The model under review builds one solid part; all positions refer to its coordinate system, in mm. A direction names the side the tool comes from. Give positions to 0.01 mm unless a question says otherwise; leave off trailing zeros. Loops run counter-clockwise (first coordinate to the right, second up) from the corner with the lowest first, then second, coordinate; pieces in that order, holes last. Notation, with made-up numbers: M 44,28.25 L 66,28.25 A21 cw 66,47.25 Z; hole C 86.25,49.5 d1. An arc over 180 degrees is marked long. Write item = value, one per line. Start each with the question number.
1. We need section A-A on y = 85.25. Give the boundary of the cut face in (x, z), then the cut area to 3 significant figures.
2. We need section C-C on y = 77.5. Give the boundary of the cut face in (x, z).
3. We need section B-B on z = 12.25. Give the boundary of the cut face in (x, y), then the cut area to 3 significant figures.
4. We need section D-D on x = 6.5. Give the boundary of the cut face in (y, z).
5. Draft analysis for pull direction Y (two halves, no side actions). For faces 1 (the face through (-6.16, 59.66, 15.14)), 2 (the face through (-15.358, 47.727, 1.479)), 3 (the face through (6, 75, 16)), state which applies: pulls with the +Y half, pulls with the -Y half, needs draft (parallel to the pull), parting line crosses it, or undercut.
6. For faces 4 (the face through (6.16, 83.54, 12.63)), 5 (the face through (0, 60, 1)), 6 (the face through (-6, 58.761, 8)), list the 3-axis set-ups (+Z, -Z, +X, -X, +Y, -Y) from which the entire face can be reached by the end or side of a thin tool; tool diameter is ignored.
7. Wall thickness on line 1 along Z through (x, y) = (6.5, 85.25); line 2 along X through (y, z) = (71, 5); line 3 along Y through (x, z) = (5.8, 12.25): over which ranges is each line inside the solid? List them lowest first. Write a range as from..to.
8. For pin 1 (5 mm diameter, centred on y = 66, z = 13, fed in from +X); pin 2 (10 mm diameter, centred on x = 8.5, z = 13, fed in from -Y); pin 3 (1.5 mm diameter, centred on y = 76.5, z = 14, fed in from -X), all flat-tipped, find the tip position at first contact; note any pin that passes through.
from build123d import *

# Parameters (mm, degrees)
SKETCH2_R           = 5
SKETCH2_R_2         = 2.75
SKETCH2_W           = 2
SKETCH2_H           = 30
BOSS_EXTRUDE1_DEPTH = 3
SKETCH3_W           = 2
SKETCH3_H           = 31.239003023
BOSS_EXTRUDE2_DEPTH = 13
SKETCH4_W           = 2
SKETCH4_H           = 29.7
BOSS_EXTRUDE3_DEPTH = 2
SKETCH5_R           = 1.75
CUT_EXTRUDE1_DEPTH  = 96.357865433
FILLET1_R           = 3


with BuildPart() as part:
    # Sketch2 → Boss-Extrude1 (new body)
    # profile 1 of 13: a face of its own
    with BuildSketch(Plane.XY):
        with BuildLine():
            Line((0, 55), (-5.15, 55))
            Line((-5.15, 55), (-7.15, 55))
            Line((-7.15, 55), (-7.15, 58.760996977))
            ThreePointArc((-7.15, 58.760996977), (-14.633199965, 54.158827301), (-19.615384615, 46.923076923))
            ThreePointArc((-19.615384615, 46.923076923), (-14.019419324, 49.902903378), (-10, 45))
            ThreePointArc((-10, 45), (-7.071067812, 52.071067812), (0, 55))
        make_face()
    # profile 2 of 13: a face of its own
    with BuildSketch(Plane.XY):
        with Locations((-15, 45)):
            Circle(SKETCH2_R)
        with Locations((-15, 45)):
            Circle(SKETCH2_R_2, mode=Mode.SUBTRACT)
    # profile 3 of 13: a face of its own
    with BuildSketch(Plane.XY):
        with BuildLine():
            Line((7.15, 55), (5.15, 55))
            Line((5.15, 55), (0, 55))
            ThreePointArc((0, 55), (7.071067812, 52.071067812), (10, 45))
            ThreePointArc((10, 45), (14.019419324, 49.902903378), (19.615384615, 46.923076923))
            ThreePointArc((19.615384615, 46.923076923), (14.633199965, 54.158827301), (7.15, 58.760996977))
            Line((7.15, 58.760996977), (7.15, 55))
        make_face()
    # profile 4 of 13: a face of its own
    with BuildSketch(Plane.XY):
        with Locations((15, 45)):
            Circle(SKETCH2_R)
        with Locations((15, 45)):
            Circle(SKETCH2_R_2, mode=Mode.SUBTRACT)
    # profile 5 of 13: a face of its own
    with BuildSketch(Plane.XY):
        with BuildLine():
            ThreePointArc((5.15, 59.366498248), (2.594408626, 59.841029939), (0, 60))
            ThreePointArc((0, 60), (-2.594408626, 59.841029939), (-5.15, 59.366498248))
            Line((-5.15, 59.366498248), (-5.15, 55))
            Line((-5.15, 55), (0, 55))
            Line((0, 55), (5.15, 55))
            Line((5.15, 55), (5.15, 59.366498248))
        make_face()
    # profile 6 of 13: a face of its own
    with BuildSketch(Plane.XY):
        with BuildLine():
            ThreePointArc((7.15, 58.760996977), (6.157447356, 59.088346591), (5.15, 59.366498248))
            Line((5.15, 59.366498248), (5.15, 55))
            Line((5.15, 55), (7.15, 55))
            Line((7.15, 55), (7.15, 58.760996977))
        make_face()
    # profile 7 of 13: a face of its own
    with BuildSketch(Plane.XY):
        with BuildLine():
            Line((-5.15, 55), (-5.15, 59.366498248))
            ThreePointArc((-5.15, 59.366498248), (-6.157447356, 59.088346591), (-7.15, 58.760996977))
            Line((-7.15, 58.760996977), (-7.15, 55))
            Line((-7.15, 55), (-5.15, 55))
        make_face()
    # profile 8 of 13: a face of its own
    with BuildSketch(Plane.XY):
        with Locations((-6.15, 75)):
            Rectangle(SKETCH2_W, SKETCH2_H)
    # profile 9 of 13: a face of its own
    with BuildSketch(Plane.XY):
        with BuildLine():
            Line((-5.15, 59.366498248), (-5.15, 60))
            Line((-5.15, 60), (-7.15, 60))
            Line((-7.15, 60), (-7.15, 58.760996977))
            ThreePointArc((-7.15, 58.760996977), (-6.157447356, 59.088346591), (-5.15, 59.366498248))
        make_face()
    # profile 10 of 13: a face of its own
    with BuildSketch(Plane.XY):
        with BuildLine():
            ThreePointArc((-5.15, 59.366498248), (-2.594408626, 59.841029939), (0, 60))
            Line((0, 60), (-5.15, 60))
            Line((-5.15, 60), (-5.15, 59.366498248))
        make_face()
    # profile 11 of 13: a face of its own
    with BuildSketch(Plane.XY):
        with BuildLine():
            Line((5.15, 60), (0, 60))
            ThreePointArc((0, 60), (2.594408626, 59.841029939), (5.15, 59.366498248))
            Line((5.15, 59.366498248), (5.15, 60))
        make_face()
    # profile 12 of 13: a face of its own
    with BuildSketch(Plane.XY):
        with BuildLine():
            Line((7.15, 60), (5.15, 60))
            Line((5.15, 60), (5.15, 59.366498248))
            ThreePointArc((5.15, 59.366498248), (6.157447356, 59.088346591), (7.15, 58.760996977))
            Line((7.15, 58.760996977), (7.15, 60))
        make_face()
    # profile 13 of 13: a face of its own
    with BuildSketch(Plane.XY):
        with Locations((6.15, 75)):
            Rectangle(SKETCH2_W, SKETCH2_H)
    extrude(amount=BOSS_EXTRUDE1_DEPTH)

    # Sketch3 → Boss-Extrude2 (add)
    with BuildSketch(Plane.XY.offset(3)):
        with Locations((-6.15, 74.380498488)):
            Rectangle(SKETCH3_W, SKETCH3_H)
        with Locations((6.15, 74.380498488)):
            Rectangle(SKETCH3_W, SKETCH3_H)
    extrude(amount=BOSS_EXTRUDE2_DEPTH)

    # Sketch4 → Boss-Extrude3 (add)
    with BuildSketch(Plane(origin=(0, 0, 0), x_dir=(-1, 0, 0), z_dir=(0, 0, -1))):
        with Locations((-6.15, 75.15)):
            Rectangle(SKETCH4_W, SKETCH4_H)
        with Locations((6.15, 75.15)):
            Rectangle(SKETCH4_W, SKETCH4_H)
    extrude(amount=BOSS_EXTRUDE3_DEPTH)

    # Sketch5 → Cut-Extrude1 (cut, through all)
    with BuildSketch(Plane(origin=(7.15, 0, 0), x_dir=(0, 0, -1), z_dir=(1, 0, 0))):
        with Locations((-1.75, 62.75)):
            Circle(SKETCH5_R)
        with Locations((-12.25, 85.25)):
            Circle(SKETCH5_R)
    extrude(amount=-CUT_EXTRUDE1_DEPTH, mode=Mode.SUBTRACT)

    # Fillet1
    # the kernel refuses this fillet: 3 mm, written as the material it takes off along each edge
    with BuildSketch(Plane(origin=(1.921067812, 60.3, -2), x_dir=(0, 0, 1), z_dir=(-1, 0, 0))) as fillet1_piece_1:
        with BuildLine():
            CenterArc((3, 2.828427125), FILLET1_R, 180, 70.528779366)
            Line((0, 2.828427125), (-0.06, 2.828427125))
            Line((-0.06, 2.828427125), (-0.06, 0))
            Line((-0.06, 0), (0, -0.06))
            ThreePointArc((0, -0.06), (1, -0.06), (1.98, -0.056568542))
            Line((1.98, -0.056568542), (2, 0))
        make_face()
    extrude(amount=16.142135624, mode=Mode.SUBTRACT)
    with BuildSketch(Plane(origin=(-1.921067812, 60.3, -2), x_dir=(0, 0, 1), z_dir=(1, 0, 0))) as fillet1_piece_2:
        with BuildLine():
            CenterArc((3, -2.828427125), FILLET1_R, 109.471220634, 70.528779366)
            Line((0, -2.828427125), (-0.06, -2.828427125))
            Line((-0.06, -2.828427125), (-0.06, 0))
            Line((-0.06, 0), (0, 0.06))
            ThreePointArc((0, 0.06), (1, 0.06), (1.98, 0.056568542))
            Line((1.98, 0.056568542), (2, 0))
        make_face()
    extrude(amount=16.142135624, mode=Mode.SUBTRACT)
    with BuildSketch(Plane(origin=(14.65, 58.760996977, 16), x_dir=(0, 0, -1), z_dir=(-1, 0, 0)), Plane(origin=(14.65, 90, -2), x_dir=(0, 0, 1), z_dir=(-1, 0, 0)), Plane(origin=(-14.65, 90, -2), x_dir=(0, -1, 0), z_dir=(1, 0, 0)), Plane(origin=(-2.35, 90, 16), x_dir=(0, 0, -1), z_dir=(1, 0, 0)), Plane(origin=(2.35, 90, 16), x_dir=(0, -1, 0), z_dir=(-1, 0, 0))) as fillet1_piece_3:
        with BuildLine():
            CenterArc((FILLET1_R, -FILLET1_R), FILLET1_R, 90, 90)
            Line((0, -FILLET1_R), (-FILLET1_R * 0.02, -FILLET1_R))
            Line((-FILLET1_R * 0.02, -FILLET1_R), (-FILLET1_R * 0.02, FILLET1_R * 0.02))
            Line((-FILLET1_R * 0.02, FILLET1_R * 0.02), (FILLET1_R, FILLET1_R * 0.02))
            Line((FILLET1_R, FILLET1_R * 0.02), (FILLET1_R, 0))
        make_face()
    extrude(amount=17, mode=Mode.SUBTRACT)
    with BuildSketch(Plane(origin=(-14.65, 58.760996977, 16), x_dir=(0, 0, -1), z_dir=(1, 0, 0))) as fillet1_piece_4:
        with BuildLine():
            CenterArc((FILLET1_R, FILLET1_R), FILLET1_R, 180, 90)
            Line((0, FILLET1_R), (-FILLET1_R * 0.02, FILLET1_R))
            Line((-FILLET1_R * 0.02, FILLET1_R), (-FILLET1_R * 0.02, -FILLET1_R * 0.02))
            Line((-FILLET1_R * 0.02, -FILLET1_R * 0.02), (FILLET1_R, -FILLET1_R * 0.02))
            Line((FILLET1_R, -FILLET1_R * 0.02), (FILLET1_R, 0))
        make_face()
    extrude(amount=17, mode=Mode.SUBTRACT)


solid = part.part
Final values:
q1.outline = M -7.15,-2 L -5.15,-2 L -5.15,10.5 L -7.15,10.5 Z; M -7.15,14 L -5.15,14 L -5.15,16 L -7.15,16 Z; M 5.15,-2 L 7.15,-2 L 7.15,10.5 L 5.15,10.5 Z; M 5.15,14 L 7.15,14 L 7.15,16 L 5.15,16 Z
q1.area = 58.0 mm²
q2.outline = M -7.15,-2 L -5.15,-2 L -5.15,16 L -7.15,16 Z; M 5.15,-2 L 7.15,-2 L 7.15,16 L 5.15,16 Z
q3.outline = M -7.15,58.76 L -5.15,58.76 L -5.15,83.5 L -7.15,83.5 Z; M -7.15,87 L -5.15,87 L -5.15,90 L -7.15,90 Z; M 5.15,58.76 L 7.15,58.76 L 7.15,83.5 L 5.15,83.5 Z; M 5.15,87 L 7.15,87 L 7.15,90 L 5.15,90 Z
q3.area = 111 mm²
q4.outline = M 52.6,0 L 60.3,0 A3 ccw 63.13,-2 L 87,-2 A3 ccw 90,1 L 90,13 A3 ccw 87,16 L 61.76,16 A3 ccw 58.76,13 L 58.76,3 L 52.6,3 Z; hole C 62.75,1.75 d3.5; hole C 85.25,12.25 d3.5
q5.face_1 = pulls with the -Y half
q5.face_2 = undercut
q5.face_3 = needs draft
q6.face_4 = +X, -X
q6.face_5 = +Z, -Z, +Y
q6.face_6 = +Z, +X, -X, -Y
q7.line_1 = -2..10.5, 14..16
q7.line_2 = -7.15..-5.15, 5.15..7.15
q7.line_3 = 58.76..83.5, 87..90
q8.pin_1 = 7.15
q8.pin_2 = 58.76
q8.pin_3 = -7.15
